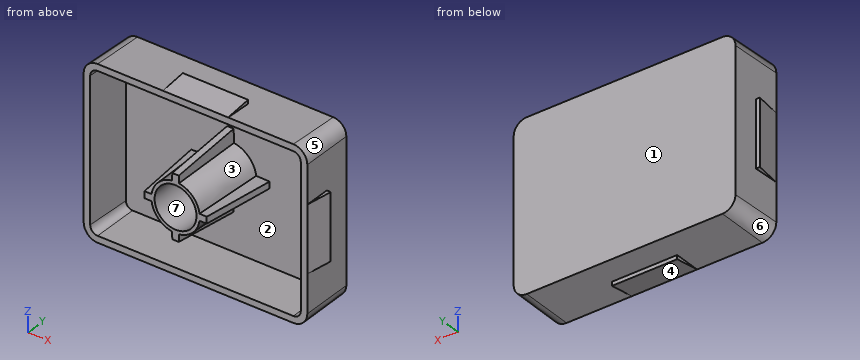
from build123d import *

# Parameters (mm, degrees)
BOSS_EXTRUDE1_DEPTH = 4
BOSS_EXTRUDE1_DRAFT = 1
SHELL1_T            = -0.5
SKETCH2_R           = 2
BOSS_EXTRUDE2_DEPTH = 5.5
BOSS_EXTRUDE2_TAPER = 1.5
CIRPATTERN1_COUNT   = 4
SKETCH4_R           = 1.605977431
CUT_EXTRUDE1_DEPTH  = 5.5
CUT_EXTRUDE1_DRAFT  = 1.5
BOSS_EXTRUDE3_DEPTH = 2.5
BOSS_EXTRUDE4_DEPTH = 2.5


with BuildPart() as part:
    # Sketch1 → Boss-Extrude1 (with draft: the straight prism first)
    with BuildSketch(Plane(origin=(0, 0, 0), x_dir=(1, 0, 0), z_dir=(0, 1, 0))):
        with BuildLine():
            Line((-7.5, -6.375), (7.5, -6.375))
            ThreePointArc((7.5, -6.375), (8.207106781, -6.082106781), (8.5, -5.375))
            Line((8.5, -5.375), (8.5, 5.375))
            ThreePointArc((8.5, 5.375), (8.207106781, 6.082106781), (7.5, 6.375))
            Line((7.5, 6.375), (-7.5, 6.375))
            ThreePointArc((-7.5, 6.375), (-8.207106781, 6.082106781), (-8.5, 5.375))
            Line((-8.5, 5.375), (-8.5, -5.375))
            ThreePointArc((-8.5, -5.375), (-8.207106781, -6.082106781), (-7.5, -6.375))
        make_face()
    extrude(amount=-BOSS_EXTRUDE1_DEPTH)
    # Boss-Extrude1: the draft: its side faces are tilted about the plane it starts from
    boss_extrude1_sides = [part.faces().sort_by_distance(p)[0] for p in [
        (0, -2, 6.375),
        (8.207106781, -2, 6.082106781),
        (8.5, -2, 0),
        (8.207106781, -2, -6.082106781),
        (0, -2, -6.375),
        (-8.207106781, -2, -6.082106781),
        (-8.5, -2, 0),
        (-8.207106781, -2, 6.082106781),
    ]]
    draft(boss_extrude1_sides, Plane(origin=(0, 0, 0), x_dir=(1, 0, 0), z_dir=(0, 1, 0)), BOSS_EXTRUDE1_DRAFT)

    # Shell1
    shell1_openings = [part.faces().sort_by_distance(p)[0] for p in [
        (0, -4, 0),
    ]]
    offset(amount=SHELL1_T, openings=shell1_openings, kind=Kind.INTERSECTION)

    # Sketch2 → Boss-Extrude2 (add)
    with BuildSketch(Plane.XZ.offset(0.5)):
        Circle(SKETCH2_R)
    extrude(amount=BOSS_EXTRUDE2_DEPTH, taper=BOSS_EXTRUDE2_TAPER)

    # Rib1: read off the stored shape, not the designer's step
    # Rib1: loft between two sections, ruled curve by curve
    rib1_from = [
        Edge.make_line((1.98200852, -0.5, 0.267660658), (3, -0.5, 0.25)),
        Edge.make_line((1.98200852, -0.5, -0.267660658), (3, -0.5, -0.25)),
        Edge.make_line((3, -0.5, -0.25), (3, -0.5, 0.25)),
        Edge.make_line((1.98200852, -0.5, -0.267660658), (1.98200852, -0.5, 0.267660658)),
    ]
    rib1_to = [
        Edge.make_line((1.837736121, -6, 0.25957306), (2.389544218, -6, 0.25)),
        Edge.make_line((1.837736121, -6, -0.25957306), (2.389544218, -6, -0.25)),
        Edge.make_line((2.389544218, -6, -0.25), (2.389544218, -6, 0.25)),
        Edge.make_line((1.837736121, -6, -0.25957306), (1.837736121, -6, 0.25957306)),
    ]
    rib1 = Solid(Shell([*[Face.make_surface_from_curves(rib1_from[k], rib1_to[k]) for k in range(4)], Face(Wire(rib1_from)), Face(Wire(rib1_to))]))
    add(rib1)

    # CirPattern1: Rib1 ×4 about axis
    cirpattern1_axis = Axis((0, 0, 0), (0, 1, 0))
    for i in range(1, CIRPATTERN1_COUNT):
        add(rib1.rotate(cirpattern1_axis, i * 360 / CIRPATTERN1_COUNT))


with BuildPart() as cut_extrude1_tool:
    # Sketch4 → Cut-Extrude1 (with draft: the straight prism first)
    with BuildSketch(Plane.XZ.offset(6)):
        Circle(SKETCH4_R)
    extrude(amount=-CUT_EXTRUDE1_DEPTH)
    # Cut-Extrude1: the draft: its side faces are tilted about the plane it starts from
    cut_extrude1_sides = [cut_extrude1_tool.faces().sort_by_distance(p)[0] for p in [
        (-1.605977431, -3.25, 0),
    ]]
    draft(cut_extrude1_sides, Plane.XZ.offset(6), CUT_EXTRUDE1_DRAFT)


with BuildPart() as part_1:
    add(part.part)

    # Cut-Extrude1: cut by cut_extrude1_tool
    add(cut_extrude1_tool.part, mode=Mode.SUBTRACT)

    # Sketch5 → Boss-Extrude3 (add, symmetric)
    with BuildSketch(Plane(origin=(0, 0, 0), x_dir=(0, 0, -1), z_dir=(1, 0, 0))):
        Polygon((6.44482026, -4), (6.40991013, -2), (6.70991013, -2), align=None)
        Polygon((-6.70991013, -2), (-6.44482026, -4), (-6.40991013, -2), align=None)
    extrude(amount=BOSS_EXTRUDE3_DEPTH, both=True)

    # Sketch6 → Boss-Extrude4 (add, symmetric)
    with BuildSketch(Plane.XY):
        Polygon((8.56982026, -4), (8.53491013, -2), (8.83491013, -2), align=None)
        Polygon((-8.83491013, -2), (-8.56982026, -4), (-8.53491013, -2), align=None)
    extrude(amount=BOSS_EXTRUDE4_DEPTH, both=True)


solid = part_1.part
Could you check a few things on this model? Use its own coordinates, in mm. Face numbers are marked on the shaded views. A direction names the side the tool comes from. Coordinates: 2 decimals unless noted, no trailing zeros. Order: outer loops, then holes, each group sorted by start corner. A loop starts at its lowest first (then second) coordinate and runs counter-clockwise, first axis right, second up.
Q1. Suppose I cut it at B-B on y = -1.25. Give the number of separate pieces and of enclosed holes in the cut face, and give its area (3 significant figures).
Q2. Thinking about a two-plate mould opening in Z: for the marked faces 1, 2, 3 and 4, which applies, released by +Z, released by -Z, zero draft, split by the parting line, or undercut?
Q3. Which directions (+Z, -Z, +X, -X, +Y, -Y) give clear straight access to the entire face, cutting with the end or side of a thin tool? Please do the marked faces 5, 6 and 7.
Q4. Please list where these lines run through material, in increasing order: L1, parallel to Z at x = -5.5, y = -3.75; L2, parallel to Z at x = 2.25, y = -3.25; L3, parallel to X at y = -1.75, z = -2.
Q5. Will these pins go through, and if not, where does the flat tip stop? pin 1 (2 mm diameter, centred on x = -4, y = -4.5, fed in from -Z); pin 2 (3 mm diameter, centred on y = -5, z = -4, fed in from +X).
Q6. Suppose I cut it at A-A on x = -5.75. Please give me the cut outline in (y, z) (3 decimals).
Answer:
1. separate pieces: 2
1. enclosed holes: 2
1. area: 33.0 mm2
2. face 1: zero draft
2. face 2: undercut
2. face 3: undercut
2. face 4: released by -Z
3. face 5: +Z, +X, +Y
3. face 6: -Z, -X, +Y
3. face 7: none
4. L1: z = -6.44 to -5.94, 5.94 to 6.44
4. L2: z = -6.54 to -5.93, -0.26 to 0.26, 5.93 to 6.54
4. L3: x = -8.53 to -8.03, -0.26 to 0.26, 8.03 to 8.53
5. pin 1: stops at z = -6.44
5. pin 2: stops at x = 8.57
6. outline: (-4, -6.445) - (0, -6.375) - (0, 6.375) - (-4, 6.445) - (-4, 5.945) - (-0.5, 5.884) - (-0.5, -5.884) - (-4, -5.945) - close
